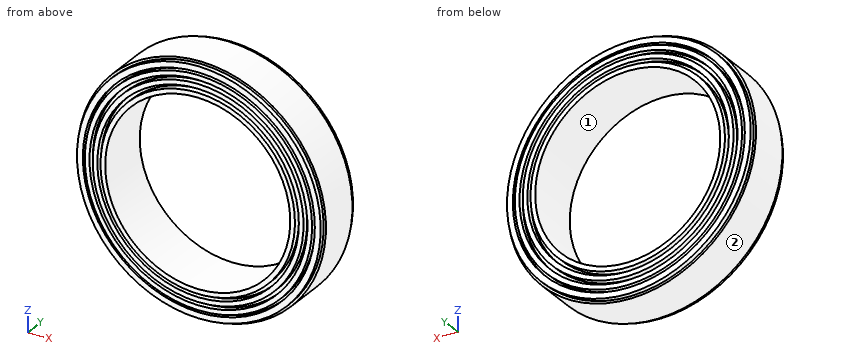
```python
from build123d import *

# Parameters (mm, degrees)
SKETCH1_R                              = 106
SKETCH1_R_2                            = 80
PRESENTATION_TIRE_CASING_ANNULUS_DEPTH = 18
SKETCH2_R                              = 104
SKETCH2_R_2                            = 99
OUTER_TIRE_SHOULDER_LINE_DEPTH         = 22
SKETCH3_R                              = 97
SKETCH3_R_2                            = 93
OUTER_TREAD_GROOVE_LINE_DEPTH          = 22.5
SKETCH4_R                              = 90
SKETCH4_R_2                            = 86
INNER_TREAD_GROOVE_LINE_DEPTH          = 23
SKETCH5_R                              = 83
SKETCH5_R_2                            = 79
INNER_TIRE_BEAD_LINE_DEPTH             = 23.5


with BuildPart() as part:
    # Sketch1 → Presentation tire casing annulus (new, symmetric)
    with BuildSketch(Plane(origin=(0, 0, 0), x_dir=(1, 0, 0), z_dir=(0, 1, 0))):
        with Locations(Location((0, 0, 0), (0, 0, 270))):
            Circle(SKETCH1_R)
        with Locations(Location((0, 0, 0), (0, 0, 270))):
            Circle(SKETCH1_R_2, mode=Mode.SUBTRACT)
    extrude(amount=PRESENTATION_TIRE_CASING_ANNULUS_DEPTH, both=True)

    # Sketch2 → outer tire shoulder line (add, symmetric)
    with BuildSketch(Plane(origin=(0, 0, 0), x_dir=(1, 0, 0), z_dir=(0, 1, 0))):
        with Locations(Location((0, 0, 0), (0, 0, 270))):
            Circle(SKETCH2_R)
        with Locations(Location((0, 0, 0), (0, 0, 270))):
            Circle(SKETCH2_R_2, mode=Mode.SUBTRACT)
    extrude(amount=OUTER_TIRE_SHOULDER_LINE_DEPTH, both=True)

    # Sketch3 → outer tread groove line (add, symmetric)
    with BuildSketch(Plane(origin=(0, 0, 0), x_dir=(1, 0, 0), z_dir=(0, 1, 0))):
        with Locations(Location((0, 0, 0), (0, 0, 90))):
            Circle(SKETCH3_R)
        with Locations(Location((0, 0, 0), (0, 0, 90))):
            Circle(SKETCH3_R_2, mode=Mode.SUBTRACT)
    extrude(amount=OUTER_TREAD_GROOVE_LINE_DEPTH, both=True)

    # Sketch4 → inner tread groove line (add, symmetric)
    with BuildSketch(Plane(origin=(0, 0, 0), x_dir=(1, 0, 0), z_dir=(0, 1, 0))):
        with Locations(Location((0, 0, 0), (0, 0, 270))):
            Circle(SKETCH4_R)
        with Locations(Location((0, 0, 0), (0, 0, 270))):
            Circle(SKETCH4_R_2, mode=Mode.SUBTRACT)
    extrude(amount=INNER_TREAD_GROOVE_LINE_DEPTH, both=True)

    # Sketch5 → inner tire bead line (add, symmetric)
    with BuildSketch(Plane(origin=(0, 0, 0), x_dir=(1, 0, 0), z_dir=(0, 1, 0))):
        with Locations(Location((0, 0, 0), (0, 0, 270))):
            Circle(SKETCH5_R)
        with Locations(Location((0, 0, 0), (0, 0, 270))):
            Circle(SKETCH5_R_2, mode=Mode.SUBTRACT)
    extrude(amount=INNER_TIRE_BEAD_LINE_DEPTH, both=True)


solid = part.part
```
Geometry: final body of the model. Coordinates: model frame, mm. Face numbers are marked on the shaded views. Round coordinates to 2 decimals unless told otherwise and drop trailing zeros. Order: outer loops, then holes, each group sorted by start corner. A loop starts at its lowest first (then second) coordinate and runs counter-clockwise, first axis right, second up. Notation, with made-up numbers: (69.5, -25) -> (106.5, -25) arc R27 cw to (106.5, 5) -> close; hole circle Ø4 at (60.25, -23.75). An arc over 180 degrees is marked (long way). Use CSV: the item, a comma, the result in double quotes. Start each with the question number.
1) First-contact query: pin 1 Ø2 at (y, z) = (-2.5, 52.5) entering from -X; pin 2 Ø6 at (y, z) = (-0.5, -17.5) entering from -X; pin 3 Ø1.5 at (x, y) = (-53.5, 6) entering from -Z. Flat tips, straight axial feed; report the tip coordinate or a pass-through.
2) Material intervals for line 1 along X through (y, z) = (4, 0); line 2 along Y through (x, z) = (-40, 83); line 3 along X through (y, z) = (12, -45), sorted ascending. Write a range as from..to.
3) Draft query along X for the marked faces 1 and 2. Return one class per face: +X half, -X half, draft (parallel to the pull), parting line (faces both ways), or undercut.
4) Section A-A (y = 3). Return the cut outline in (x, z).
Returned:
1,pin 1,"stops at x = -92.65"
1,pin 2,"stops at x = -105"
1,pin 3,"stops at z = -91.94"
2,line 1,"x = -106..-79, 79..106"
2,line 2,"y = -18..18"
2,line 3,"x = -95.97..-64.93, 64.93..95.97"
3,face 1,"undercut"
3,face 2,"parting line"
4,outline,"circle Ø212 at (0, 0); hole circle Ø158 at (0, 0)"
